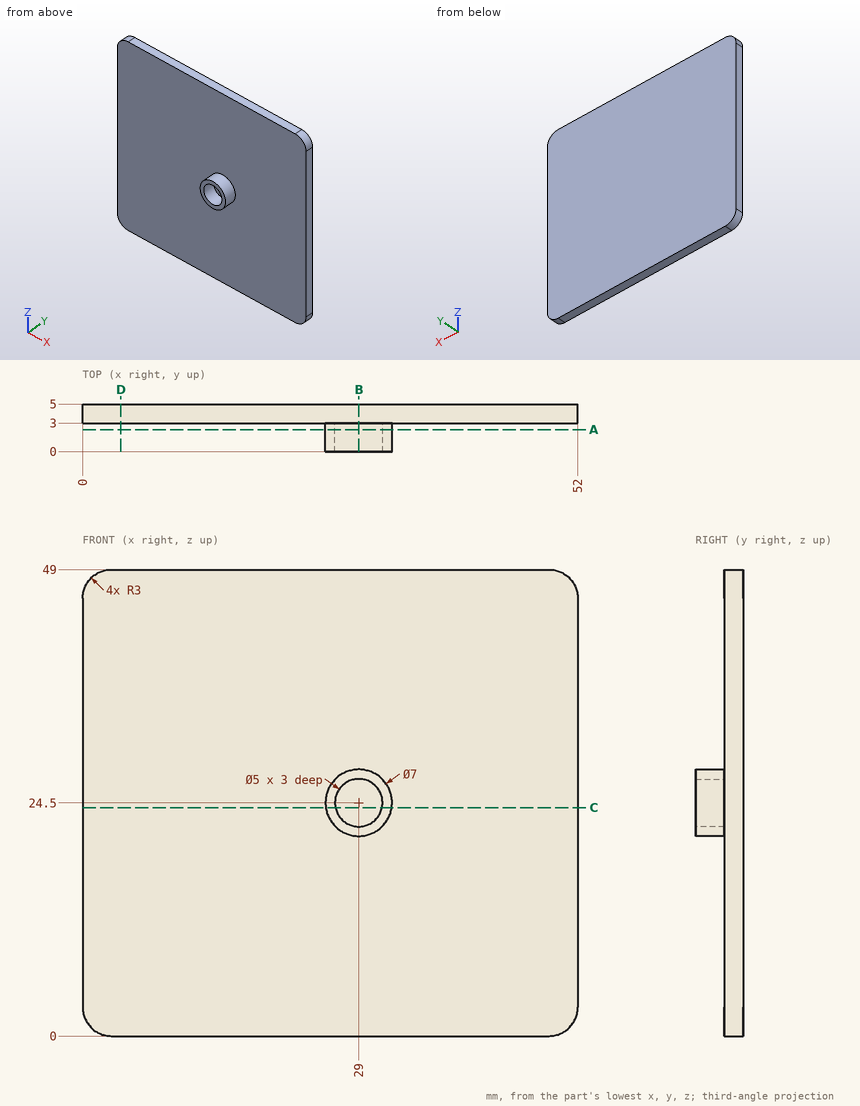
Drawing for the job (mm, zero at the part's lowest x, y, z). Give positions to 0.01 mm unless a question says otherwise; leave off trailing zeros. Loops run counter-clockwise (first coordinate to the right, second up) from the corner with the lowest first, then second, coordinate; pieces in that order, holes last.
Item 1: Slice it at D-D (x = 4). Write the cut outline in (y, z), plus the area to 3 significant figures.
Check values:
outline: (3, 0) - (5, 0) - (5, 49) - (3, 49) - close
area: 98.0 mm2
Item 2: Drop flat-ended pins along their axis: P1, Ø4, axis at x = 25, z = 18.5, coming from the -Y side; P2, Ø3, axis at y = 2, z = 7, coming from the +X side. Give the stop position or say it passes through.
Check values:
P1: stops at y = 3
P2: stops at x = 52
Item 3: Slice it at A-A (y = 2.3). Write the cut outline in (x, z), plus the area to 3 significant figures.
Check values:
outline: circle Ø7 at (29, 24.5); hole circle Ø5 at (29, 24.5)
area: 18.8 mm2
Item 4: Slice it at B-B (x = 29). Write the cut outline in (y, z).
Check values:
outline: (0, 21) - (3, 21) - (3, 0) - (5, 0) - (5, 49) - (3, 49) - (3, 28) - (0, 28) - (0, 27) - (3, 27) - (3, 22) - (0, 22) - close
Item 5: Drill centre lines: line 1 along X through (y, z) = (1.8, 24.5); line 2 along Y through (x, z) = (16, 45); line 3 along Z through (x, y) = (29.5, 2.1). Where is each one in solid material? Low to high.
Check values:
line 1: x = 25.5 to 26.5, 31.5 to 32.5
line 2: y = 3 to 5
line 3: z = 21.04 to 22.05, 26.95 to 27.96
Item 6: Slice it at C-C (z = 24). Write the cut outline in (x, y).
Check values:
outline: (0, 3) - (25.54, 3) - (25.54, 0) - (26.55, 0) - (26.55, 3) - (31.45, 3) - (31.45, 0) - (32.46, 0) - (32.46, 3) - (52, 3) - (52, 5) - (0, 5) - close
